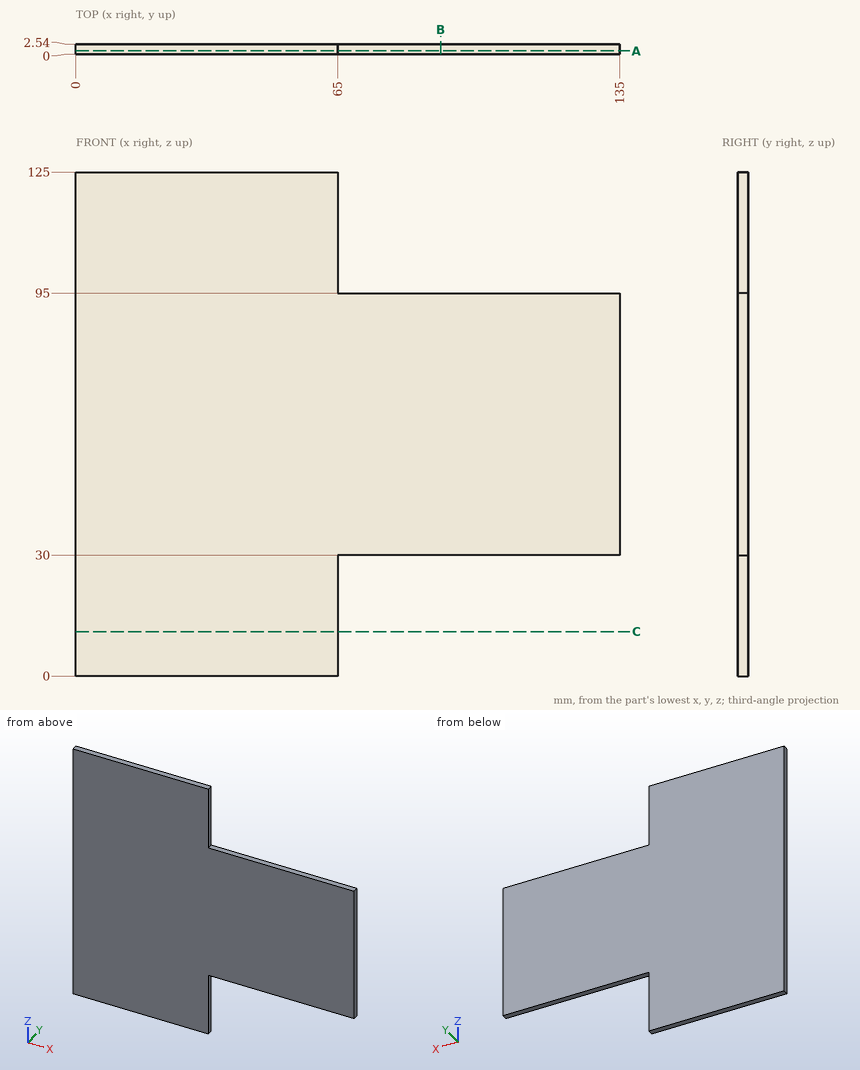
Can you work these out from the drawing? Everything is in mm from the part's minimum corner. Round coordinates to 2 decimals unless told otherwise and drop trailing zeros. Order: outer loops, then holes, each group sorted by start corner. A loop starts at its lowest first (then second) coordinate and runs counter-clockwise, first axis right, second up. Notation, with made-up numbers: (4, 36) - (60, 36) arc R35 cw to (60, 75) - close; hole circle Ø4 at (-23.75, 19.25). An arc over 180 degrees is marked (long way). Answer in a Markdown table with one row per item.
(1) Suppose I cut it at A-A, the plane y = 0.85. Please give me the cut outline in (x, z), plus the area to 3 significant figures.
From the geometry:
| item | result |
|---|---|
| outline | (0, 0) - (65, 0) - (65, 30) - (135, 30) - (135, 95) - (65, 95) - (65, 125) - (0, 125) - close |
| area | 12,700 mm2 |
(2) For P1, Ø0.8, axis at y = 2, z = 10.5, coming from the +X side; P2, Ø1.3, axis at x = 83, y = 0.5, coming from the -Z side, each with a flat end and sliding along its axis, tell me the tip position at first contact or that it passes through.
From the geometry:
| item | result |
|---|---|
| P1 | stops at x = 65 |
| P2 | stops at z = 30 |
(3) Please list where these lines run through material, in increasing order: L1, parallel to Z at x = 74, y = 1.55; L2, parallel to X at y = 2.2, z = 19. Write a range as from..to.
From the geometry:
| item | result |
|---|---|
| L1 | z = 30..95 |
| L2 | x = 0..65 |
(4) Suppose I cut it at C-C, the plane z = 11. Please give me the cut outline in (x, y), plus the area to 3 significant figures.
From the geometry:
| item | result |
|---|---|
| outline | (0, 0) - (65, 0) - (65, 2.54) - (0, 2.54) - close |
| area | 165 mm2 |
(5) Suppose I cut it at B-B, the plane x = 90.5. Please give me the cut outline in (y, z).
From the geometry:
| item | result |
|---|---|
| outline | (0, 30) - (2.54, 30) - (2.54, 95) - (0, 95) - close |
